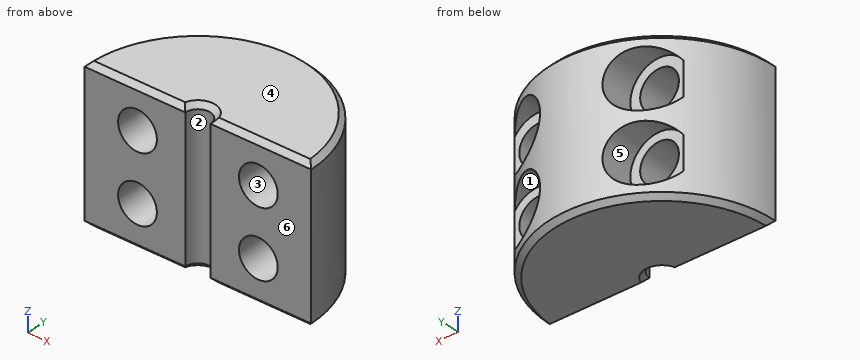
from build123d import *

# Parameters (mm, degrees)
BOSS_EXTRUDE2_DEPTH = 15.24
CHAMFER1_SIZE       = 0.508
SKETCH4_R           = 2.9464
SKETCH4_R_2         = 1.9558
CUT_EXTRUDE1_DEPTH  = 3.81
SKETCH6_R           = 1.9558
CUT_EXTRUDE2_DEPTH  = 12.4300001


with BuildPart() as part:
    # Sketch2 → Boss-Extrude2 (new body)
    with BuildSketch(Plane.XY):
        with BuildLine():
            Line((-11.43, 0), (-1.27, 0))
            ThreePointArc((-1.27, 0), (0, 1.27), (1.27, 0))
            Line((1.27, 0), (11.43, 0))
            ThreePointArc((11.43, 0), (0, 11.43), (-11.43, 0))
        make_face()
    extrude(amount=BOSS_EXTRUDE2_DEPTH)

    # Chamfer1
    chamfer1_edges = [part.edges().sort_by_distance(p)[0] for p in [
        (0, 11.43, 15.24),
        (-6.35, 0, 15.24),
        (0, 1.27, 15.24),
        (-6.35, 0, 0),
        (0, 11.43, 0),
        (6.35, 0, 0),
        (0, 1.27, 0),
        (6.35, 0, 15.24),
    ]]
    chamfer(chamfer1_edges, length=CHAMFER1_SIZE)

    # Sketch4 → Cut-Extrude1 (cut)
    with BuildSketch(Plane(origin=(0, 11.43, 0), x_dir=(1, 0, 0), z_dir=(0, 1, 0))):
        with Locations((-6.096, -4.191)):
            Circle(SKETCH4_R)
        with Locations((-6.096, -4.303195449)):
            Circle(SKETCH4_R_2, mode=Mode.SUBTRACT)
        with Locations((-6.096, -11.049)):
            Circle(SKETCH4_R)
        with Locations((-6.096, -11.049)):
            Circle(SKETCH4_R_2, mode=Mode.SUBTRACT)
        with Locations((6.096, -4.191)):
            Circle(SKETCH4_R)
        with Locations((6.096, -4.303195449)):
            Circle(SKETCH4_R_2, mode=Mode.SUBTRACT)
        with Locations((6.096, -11.049)):
            Circle(SKETCH4_R)
        with Locations((6.096, -11.049)):
            Circle(SKETCH4_R_2, mode=Mode.SUBTRACT)
    extrude(amount=-CUT_EXTRUDE1_DEPTH, mode=Mode.SUBTRACT)

    # Sketch6 → Cut-Extrude2 (cut, through all)
    with BuildSketch(Plane(origin=(0, 11.43, 0), x_dir=(1, 0, 0), z_dir=(0, 1, 0))):
        with Locations((-6.096, -4.303195449)):
            Circle(SKETCH6_R)
        with Locations((-6.096, -11.049)):
            Circle(SKETCH6_R)
        with Locations((6.096, -11.049)):
            Circle(SKETCH6_R)
        with Locations((6.096, -4.303195449)):
            Circle(SKETCH6_R)
    extrude(amount=-CUT_EXTRUDE2_DEPTH, mode=Mode.SUBTRACT)


solid = part.part
Geometry check sheet. Reference: the model listing, model coordinates, mm. Face numbers are marked on the shaded views. A direction names the side the tool comes from. Round coordinates to 2 decimals unless told otherwise and drop trailing zeros. Order: outer loops, then holes, each group sorted by start corner. A loop starts at its lowest first (then second) coordinate and runs counter-clockwise, first axis right, second up. Notation, with made-up numbers: (-6, 34) -> (49, 34) arc R35 ccw to (49, 67) -> close; hole circle Ø2 at (-13, 28). An arc over 180 degrees is marked (long way). Use one line per item in the form item = value.
1. Cross-section at C-C, the plane z = 8.5. Enter the section's corners in (x, y), plus the area to 3 significant figures.
Working result:
outline = (-11.43, 0) -> (-1.27, 0) arc R1.27 cw to (1.27, 0) -> (11.43, 0) arc R11.43 ccw to (7.57, 8.56) -> (7.57, 7.62) -> (4.62, 7.62) -> (4.62, 10.46) arc R11.43 ccw to (-4.62, 10.46) -> (-4.62, 7.62) -> (-7.57, 7.62) -> (-7.57, 8.56) arc R11.43 ccw to start
area = 191 mm^2
2. Mould release check, pull along Z, two halves, no side actions. Record for the marked faces 3, 4, 5 and 6: pulls with the +Z half, pulls with the -Z half, needs draft (parallel to the pull), parting line crosses it, or undercut.
Working result:
face_3 = undercut
face_4 = pulls with the +Z half
face_5 = undercut
face_6 = needs draft
3. Cross-section at A-A, the plane x = 0. Enter the section's corners in (y, z), plus the area to 3 significant figures.
Working result:
outline = (1.27, 0.51) -> (1.78, 0) -> (10.92, 0) -> (11.43, 0.51) -> (11.43, 14.73) -> (10.92, 15.24) -> (1.78, 15.24) -> (1.27, 14.73) -> close
area = 154 mm^2
4. Set-up check for the marked faces 1 and 2: record each of +Z, -Z, +X, -X, +Y, -Y from which the full face is reachable in a straight line by a thin tool's end or side.
Working result:
face_1 = +Y
face_2 = +Z, -Z, -Y
5. Cross-section at B-B, the plane y = 0.75. Count the separate pieces of the cut face and the enclosed holes in it, plus the area to 3 significant figures.
Working result:
separate_pieces = 2
enclosed_holes = 4
area = 267 mm^2
6. Go/stop test with flat-tipped pins: pin 1 (4.5 mm diameter, centred on x = -5, z = 5, fed in from +Y); pin 2 (4.5 mm diameter, centred on x = -6.096, z = 4.191, fed in from +Y); pin 3 (2.5 mm diameter, centred on x = -6.096, z = 11.049, fed in from -Y); pin 4 (3 mm diameter, centred on y = 9.5, z = 4.5, fed in from -X). Record where each tip stops, or that it passes through.
Working result:
pin_1 = 11.09
pin_2 = 7.62
pin_3 = through
pin_4 = -3.77
7. Scan lines: line 1 along Z through (x, y) = (7.25, 4.5); line 2 along X through (y, z) = (2, 11.5); line 3 along Z through (x, y) = (5, 5.5). Record each from-to range of solid material in increasing order. Write a range as from..to.
Working result:
line_1 = 0..2.72, 5.88..9.47, 12.63..15.24
line_2 = -11.25..-8, -4.19..4.19, 8..11.25
line_3 = 0..2.68, 5.92..9.43, 12.67..15.24
